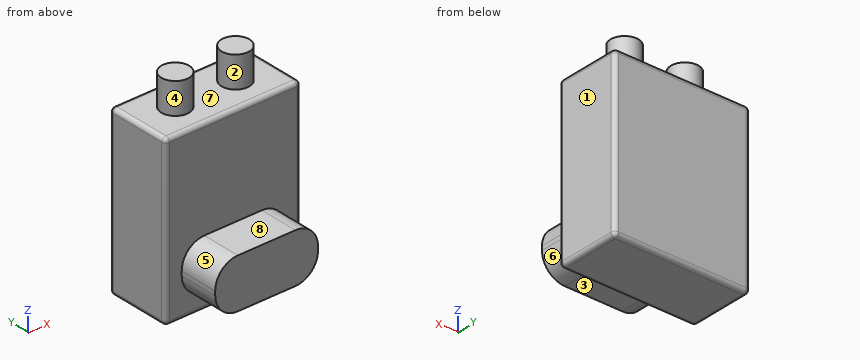
from build123d import *

# Parameters (mm, degrees)
SKETCH1_W           = 66
SKETCH1_H           = 80.5
BOSS_EXTRUDE1_DEPTH = 24.14
SKETCH2_W           = 50
SKETCH2_H           = 24
BOSS_EXTRUDE2_DEPTH = 19
SKETCH3_W           = 66
SKETCH3_H           = 80.5
BOSS_EXTRUDE3_DEPTH = 7.3
FILLET1_R           = 2
FILLET2_R           = 11
SKETCH4_R           = 6.75
BOSS_EXTRUDE4_DEPTH = 15


with BuildPart() as part:
    # Sketch1 → Boss-Extrude1 (new body)
    with BuildSketch(Plane(origin=(0, 0, 0), x_dir=(1, 0, 0), z_dir=(0, 1, 0))):
        Rectangle(SKETCH1_W, SKETCH1_H)
    extrude(amount=BOSS_EXTRUDE1_DEPTH)

    # Sketch2 → Boss-Extrude2 (add)
    with BuildSketch(Plane.XZ):
        with Locations((0, -20.25)):
            Rectangle(SKETCH2_W, SKETCH2_H)
    extrude(amount=BOSS_EXTRUDE2_DEPTH)

    # Sketch3 → Boss-Extrude3 (add)
    with BuildSketch(Plane(origin=(0, 24.14, 0), x_dir=(1, 0, 0), z_dir=(0, 1, 0))):
        Rectangle(SKETCH3_W, SKETCH3_H)
    extrude(amount=BOSS_EXTRUDE3_DEPTH)

    # Fillet1
    fillet1_edges = [part.edges().sort_by_distance(p)[0] for p in [
        (0, 31.44, 40.25),
        (33, 31.44, 0),
        (0, 31.44, -40.25),
        (-33, 31.44, 0),
        (0, 0, 40.25),
        (-33, 0, 0),
        (0, 0, -40.25),
        (33, 0, 0),
        (33, 15.72, 40.25),
        (-33, 15.72, 40.25),
        (-33, 15.72, -40.25),
        (33, 15.72, -40.25),
    ]]
    fillet(fillet1_edges, radius=FILLET1_R)

    # Fillet2
    fillet2_edges = [part.edges().sort_by_distance(p)[0] for p in [
        (-25, -9.5, -8.25),
        (-25, -9.5, -32.25),
        (25, -9.5, -32.25),
        (25, -9.5, -8.25),
    ]]
    fillet(fillet2_edges, radius=FILLET2_R)

    # Sketch4 → Boss-Extrude4 (add)
    with BuildSketch(Plane.XY.offset(40.25)):
        with Locations(Location((-14.64999991, 15.7200005, 0), (0, 0, 180))):
            Circle(SKETCH4_R)
        with Locations(Location((14.64999991, 15.7200005, 0), (0, 0, 180))):
            Circle(SKETCH4_R)
    extrude(amount=BOSS_EXTRUDE4_DEPTH)


solid = part.part
Source: CAD feature listing. Evaluate the final solid. Frame: model axes, mm. Face numbers are marked on the shaded views. A direction names the side the tool comes from. Round coordinates to 2 decimals unless told otherwise and drop trailing zeros. Loops run counter-clockwise (first coordinate to the right, second up) from the corner with the lowest first, then second, coordinate; pieces in that order, holes last. Notation, with made-up numbers: (-23.5, 15) -> (-9.5, 15) arc R16 ccw to (-9.5, 41) -> close; hole circle Ø6 at (20, -17.5). An arc over 180 degrees is marked (long way). Answer as a JSON object with one key per item and string values. Group by question number.
Q1. Section query C-C (z = 43). Output: boundary loops of the cut face in (x, y), plus the area to 3 significant figures.
Q2. Mould query, pull axis X, two halves, no side actions, for the marked faces 1, 2, 3 and 4. Classes: pulls with the +X half, pulls with the -X half, needs draft (parallel to the pull), parting line crosses it, or undercut.
Q3. Section query B-B (y = -13). Output: boundary loops of the cut face in (x, z).
Q4. Contact query for flat-ended pins moving along their axis: P1, Ø1, axis at y = -12.5, z = -20, coming from the +X side; P2, Ø5.5, axis at x = -1.5, y = -8, coming from the +Z side; P3, Ø9.5, axis at x = 3.5, y = -12.5, coming from the -Z side. Output: stop coordinate, or through.
Q5. Ray query, line 1 (Y direction, x = -18, z = 8.5); line 2 (Z direction, x = -5, y = 10.5); line 3 (X direction, y = 11, z = 42). Return the intervals inside material, ascending. Write a range as from..to.
Q6. Section query D-D (z = -24.5). Output: boundary loops of the cut face in (x, y).
Q7. Section query A-A (x = 28.5). Output: boundary loops of the cut face in (y, z).
Q8. Access query for the marked faces 5, 6, 7 and 8. Directions: +Z, -Z, +X, -X, +Y, -Y. A direction counts if a zero-diameter tool reaches every point of the face in a straight line with its end or side. Return the directions, or none.
Completed:
{
 "1": {"outline": "circle Ø13.5 at (-14.65, 15.72); circle Ø13.5 at (14.65, 15.72)", "area": "286 mm²"},
 "2": {"face 1": "pulls with the +X half", "face 2": "undercut", "face 3": "needs draft", "face 4": "undercut"},
 "3": {"outline": "(-25, -21.25) arc R11 ccw to (-14, -32.25) -> (14, -32.25) arc R11 ccw to (25, -21.25) -> (25, -19.25) arc R11 ccw to (14, -8.25) -> (-14, -8.25) arc R11 ccw to (-25, -19.25) -> close"},
 "4": {"P1": "x = 25", "P2": "z = -8.25", "P3": "z = -32.25"},
 "5": {"line 1": "0..31.44", "line 2": "-40.25..40.25", "line 3": "-19.48..-9.82, 9.82..19.48"},
 "6": {"outline": "(-33, 2) arc R2 ccw to (-31, 0) -> (-24.51, 0) -> (-24.51, -19) -> (24.51, -19) -> (24.51, 0) -> (31, 0) arc R2 ccw to (33, 2) -> (33, 29.44) arc R2 ccw to (31, 31.44) -> (-31, 31.44) arc R2 ccw to (-33, 29.44) -> close"},
 "7": {"outline": "(0, -38.25) arc R2 ccw to (2, -40.25) -> (29.44, -40.25) arc R2 ccw to (31.44, -38.25) -> (31.44, 38.25) arc R2 ccw to (29.44, 40.25) -> (2, 40.25) arc R2 ccw to (0, 38.25) -> close"},
 "8": {"face 5": "+Z, -X, -Y", "face 6": "-Z, +X, -Y", "face 7": "+Z", "face 8": "+Z, +X, -X, -Y"}
}
